For this review, use the dimensioned drawing (mm, ordinates from the lowest corner) and the shaded views. Coordinates: 2 decimals unless noted, no trailing zeros. Order: outer loops, then holes, each group sorted by start corner. A loop starts at its lowest first (then second) coordinate and runs counter-clockwise, first axis right, second up. Notation, with made-up numbers: (-7.5, 27.5) -> (34.5, 27.5) arc R30 ccw to (34.5, 59.5) -> close; hole circle Ø2 at (-21.5, 37). An arc over 180 degrees is marked (long way). Use CSV: the item, a comma, the result in double quotes. Start each with the question number.
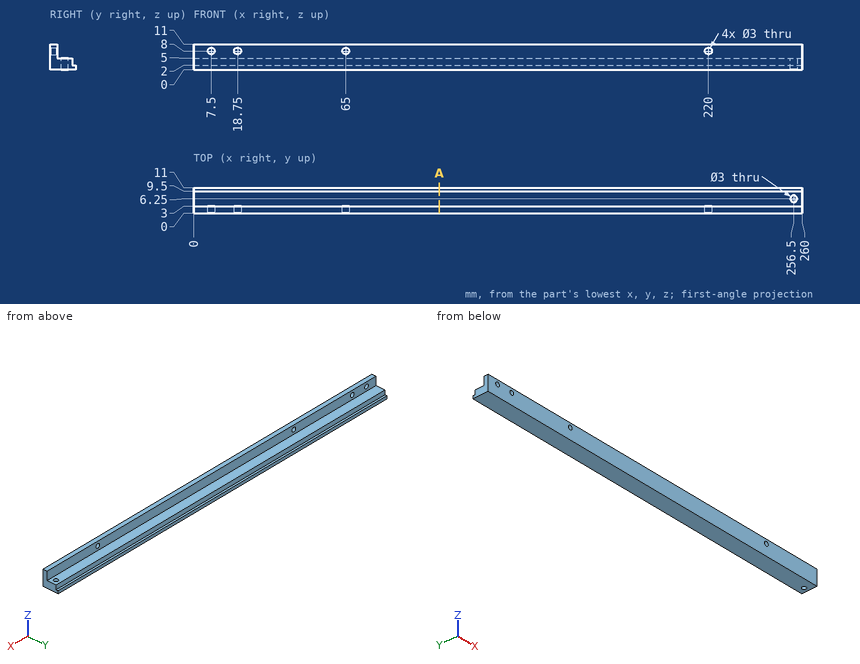
Q1. Add section A-A, the plane x = 105. State the section outline as (y, z) points.
Q2. Clearance check with flat-ended pins moving along their axes: pin 1 Ø4 at (x, z) = (122, 4.5) entering from +Y; pin 2 Ø4 at (x, z) = (65, 8) entering from +Y; pin 3 Ø3 at (x, y) = (102.5, 6.5) entering from +Z. State where each tip first meets the part, or that it passes through.
Q3. To check wall thickness, follow probe 1 along X at (y, z) = (0.9, 8); probe 2 along Z at (x, y) = (18.75, 1.9); probe 3 along Z at (x, y) = (164, 8.5). State the ranges of each line that lie inside material, in increasing order.
Answer block:
1,outline,"(0, 0) -> (11, 0) -> (11, 2) -> (9.5, 2) -> (9.5, 5) -> (3, 5) -> (3, 11) -> (0, 11) -> close"
2,pin 1,"stops at y = 9.5"
2,pin 2,"stops at y = 3"
2,pin 3,"stops at z = 5"
3,probe 1,"x = 0 to 6, 9 to 17.25, 20.25 to 63.5, 66.5 to 218.5, 221.5 to 260"
3,probe 2,"z = 0 to 6.5, 9.5 to 11"
3,probe 3,"z = 0 to 5"
